from build123d import *

# Parameters (mm, degrees)
F0_R     = 1.65
F1_DEPTH = 3
F3_DEPTH = 2.5


with BuildPart() as f1:
    # F0 (on Front) → F1 (new body)
    with BuildSketch(Plane.XZ):
        with BuildLine():
            ThreePointArc((-8.5, 13), (-10.267767, 13.732233), (-11, 15.5))
            ThreePointArc((-11, 15.5), (-15.5, 20), (-20, 15.5))
            Line((-20, 15.5), (-20, -15.5))
            ThreePointArc((-20, -15.5), (-15.5, -20), (-11, -15.5))
            ThreePointArc((-11, -15.5), (-10.267767, -13.732233), (-8.5, -13))
            Line((-8.5, -13), (8.5, -13))
            ThreePointArc((8.5, -13), (10.267767, -13.732233), (11, -15.5))
            ThreePointArc((11, -15.5), (15.5, -20), (20, -15.5))
            Line((20, -15.5), (20, 15.5))
            ThreePointArc((20, 15.5), (15.5, 20), (11, 15.5))
            ThreePointArc((11, 15.5), (10.267767, 13.732233), (8.5, 13))
            Line((8.5, 13), (-8.5, 13))
        make_face()
        with Locations((-15.5, -15.5)):
            Circle(F0_R, mode=Mode.SUBTRACT)
        with Locations((15.5, -15.5)):
            Circle(F0_R, mode=Mode.SUBTRACT)
        with BuildLine():
            Line((-8.5, -3), (8.5, -3))
            ThreePointArc((8.5, -3), (10.267767, -3.732233), (11, -5.5))
            Line((11, -5.5), (11, -6.5))
            ThreePointArc((11, -6.5), (10.267767, -8.267767), (8.5, -9))
            Line((8.5, -9), (-8.5, -9))
            ThreePointArc((-8.5, -9), (-10.267767, -8.267767), (-11, -6.5))
            Line((-11, -6.5), (-11, -5.5))
            ThreePointArc((-11, -5.5), (-10.267767, -3.732233), (-8.5, -3))
        make_face(mode=Mode.SUBTRACT)
        with Locations((-15.5, 15.5)):
            Circle(F0_R, mode=Mode.SUBTRACT)
        with BuildLine():
            ThreePointArc((11, 5.5), (10.267767, 3.732233), (8.5, 3))
            Line((8.5, 3), (-8.5, 3))
            ThreePointArc((-8.5, 3), (-10.267767, 3.732233), (-11, 5.5))
            Line((-11, 5.5), (-11, 6.5))
            ThreePointArc((-11, 6.5), (-10.267767, 8.267767), (-8.5, 9))
            Line((-8.5, 9), (8.5, 9))
            ThreePointArc((8.5, 9), (10.267767, 8.267767), (11, 6.5))
            Line((11, 6.5), (11, 5.5))
        make_face(mode=Mode.SUBTRACT)
        with Locations((15.5, 15.5)):
            Circle(F0_R, mode=Mode.SUBTRACT)
    extrude(amount=F1_DEPTH)

    # F2 (on face) → F3 (join)
    with BuildSketch(Plane.XZ.offset(3)):
        with BuildLine():
            Line((8.5, -10), (-8.5, -10))
            ThreePointArc((-8.5, -10), (-10, -11.5), (-8.5, -13))
            Line((-8.5, -13), (8.5, -13))
            ThreePointArc((8.5, -13), (10, -11.5), (8.5, -10))
        make_face()
        with BuildLine():
            ThreePointArc((-8.5, 13), (-10, 11.5), (-8.5, 10))
            Line((-8.5, 10), (8.5, 10))
            ThreePointArc((8.5, 10), (10, 11.5), (8.5, 13))
            Line((8.5, 13), (-8.5, 13))
        make_face()
    extrude(amount=F3_DEPTH)


solid = f1.part
CAD build for the part. Positions are in the model's coordinates, mm. A direction names the side the tool comes from. Round coordinates to 2 decimals unless told otherwise and drop trailing zeros. Loops run counter-clockwise (first coordinate to the right, second up) from the corner with the lowest first, then second, coordinate; pieces in that order, holes last. Notation, with made-up numbers: (10.25, 68.25) - (21.25, 68.25) arc R8 cw to (21.25, 78.25) - close; hole circle Ø7 at (77.25, 67.5). An arc over 180 degrees is marked (long way). Put each result on its own line as item: value.
1. 3-axis set-ups, long thin cutter, end or side, ignore diameter. For faces 1 (the flat face through (0, -4, -10)), 2 (the flat face through (0, -1, 3)), 3 (the cylindrical face through (-10.287, -1.479, -13.752)): which of +Z, -Z, +X, -X, +Y, -Y reach the whole face in a straight line?
Geometry check:
face 1: +X, -X, -Y
face 2: +Y, -Y
face 3: -Z, +Y, -Y
2. Pin check, flat tips, straight feed: P1, Ø0.8, axis at x = 1.5, y = -3.5, coming from the -Z side; P2, Ø0.8, axis at x = -1, y = -4.5, coming from the +Z side; P3, Ø12, axis at x = 8.5, z = 1, coming from the -Y side. Stop position of each tip, or through.
Geometry check:
P1: z = -13
P2: z = 13
P3: y = -3
3. Wall check: line 1 (Z direction, x = 15.5, y = -0.65); line 2 (Z direction, x = 6.5, y = -0.9); line 3 (X direction, y = -2.75, z = 6.5). Give the ranges that are in metal, low to high.
Geometry check:
line 1: -20 to -17.15, -13.85 to 13.85, 17.15 to 20
line 2: -13 to -9, -3 to 3, 9 to 13
line 3: -20 to -11, 11 to 20
4. Slice it at D-D on z = -11.5. List the corners of the cut face in (x, y).
Geometry check:
outline: (-20, -3) - (-10, -3) - (-10, -5.5) - (10, -5.5) - (10, -3) - (20, -3) - (20, 0) - (-20, 0) - close
5. Slice it at B-B on y = -3.7. List the corners of the cut face in (x, z).
Geometry check:
outline: (-8.5, -13) - (8.5, -13) arc R1.5 ccw to (8.5, -10) - (-8.5, -10) arc R1.5 ccw to start; (-8.5, 10) - (8.5, 10) arc R1.5 ccw to (8.5, 13) - (-8.5, 13) arc R1.5 ccw to start
6. Slice it at A-A on z = 8. List the corners of the cut face in (x, y).
Geometry check:
outline: (-20, -3) - (-10.5, -3) - (-10.5, 0) - (-20, 0) - close; (10.5, -3) - (20, -3) - (20, 0) - (10.5, 0) - close
7. Slice it at C-C on x = -14.5. List the corners of the cut face in (y, z), and give its area (3 significant figures).
Geometry check:
outline: (-3, -19.89) - (0, -19.89) - (0, -16.81) - (-3, -16.81) - close; (-3, -14.19) - (0, -14.19) - (0, 14.19) - (-3, 14.19) - close; (-3, 16.81) - (0, 16.81) - (0, 19.89) - (-3, 19.89) - close
area: 104 mm²
8. Two-plate mould, pull along X, no slides. Class faces 4 (the flat face through (0, -3, 0)), 5 (the cylindrical face through (-10, -4.2, 11.5)), 6 (the cylindrical face through (10.248, -1.479, 8.287)): released by +X, released by -X, zero draft, split by the parting line, or undercut.
Geometry check:
face 4: zero draft
face 5: released by -X
face 6: undercut
